Autodesk Inventor part; units mm, degrees
ref_plane "Work Plane1" through (47.9215, -19.8251, -5.5) normal (0, 0, 1) x (1, 0, 0)
ref_plane "Work Plane2" through (55.1914, -9.495, -5.5) normal (0, 0, 1) x (1, 0, 0)
ref_plane "YZ Plane" through (0, 0, 0) normal (1, 0, 0) x (0, 1, 0)
sketch "Sketch1" plane through (0, 0, 0) normal (0, 0, 1) x (1, 0, 0)
  circle A0 centre (66.3461, 11.6829) radius 1.35
  circle A1 centre (66.349, 28.6829) radius 1.35
  circle A2 centre (72.6461, 5.1829) radius 1.35
  circle A3 centre (72.649, 35.1829) radius 1.35
  line L0 (77.149, 32.3829) -> (77.149, 37.9829)
  line L1 (77.149, 7.9829) -> (77.149, 2.3829)
  line L2 (77.149, 32.3829) -> (69.149, 32.3829)
  line L3 (69.149, 32.3829) -> (69.149, 7.9829)
  line L4 (69.149, 7.9829) -> (77.149, 7.9829)
  circle A4 centre (16.149, 20.1829) radius 4.5
  line L5 (77.149, 37.9829) -> (52.149, 37.9829)
  arc A5 (14.1608, 31.0018) -> (14.1608, 9.3641) centre (16.149, 20.1829) ccw
  line L6 (52.149, 37.9829) -> (14.1608, 31.0018)
  line L7 (77.149, 2.3829) -> (52.149, 2.3829)
  line L8 (52.149, 2.3829) -> (14.1608, 9.3641)
  line L9 (63.549, 7.9829) -> (63.549, 32.3829)
  line L10 (63.549, 32.3829) -> (52.149, 32.3829)
  line L11 (52.149, 32.3829) -> (24.5301, 27.3073)
  line L12 (52.149, 7.9829) -> (63.549, 7.9829)
  line L13 (52.149, 7.9829) -> (24.5301, 13.0585)
  arc A6 (24.5301, 13.0585) -> (24.5301, 27.3073) centre (16.149, 20.1829) ccw
  point P0 (0, 0)
  dimension "d2" = 9
  dimension "d26" = 8
  dimension "d27" = 8
  dimension "d29" = 2.8
  dimension "d30" = 6.3
  dimension "d31" = 6.3
  dimension "d32" = 25
  dimension "d33" = 22
  dimension "d34" = 25
  dimension "d43" = 5.6
  dimension "d44" = 5.6
  dimension "d46" = 5.6
  dimension "d47" = 11.4
  dimension "d48" = 11.4
extrude "Extrusion1" add sketch "Sketch1" along normal blind 3
ref_plane "Work Plane1" through (47.9215, -19.8251, -5.5) normal (0, 0, 1) x (1, 0, 0)
sketch "Sketch5" plane through (0, 0, 0) normal (0, 0, -1) x (-1, 0, 0)
  line L0 (-52.149, 7.9829) -> (-63.549, 7.9829)
  line L1 (-63.549, 32.3829) -> (-52.149, 32.3829)
  circle A0 centre (-72.6461, 5.1829) radius 1.35
  circle A1 centre (-66.349, 28.6829) radius 1.35
  circle A2 centre (-66.3461, 11.6829) radius 1.35
  circle A3 centre (-72.649, 35.1829) radius 1.35
  line L2 (-77.149, 32.3829) -> (-77.149, 37.9829)
  line L3 (-77.149, 2.3829) -> (-77.149, 7.9829)
  line L4 (-77.149, 37.9829) -> (-52.149, 37.9829)
  line L5 (-77.149, 32.3829) -> (-69.149, 32.3829)
  line L6 (-69.149, 32.3829) -> (-69.149, 7.9829)
  line L7 (-69.149, 7.9829) -> (-77.149, 7.9829)
  line L8 (-77.149, 7.9829) -> (-77.149, 2.3829)
  line L9 (-77.149, 2.3829) -> (-52.149, 2.3829)
  line L10 (-52.149, 2.3829) -> (-52.149, 7.9829)
  line L11 (-63.549, 7.9829) -> (-63.549, 32.3829)
  line L12 (-52.149, 32.3829) -> (-52.149, 37.9829)
  line L13 (-63.549, 32.3829) -> (-52.149, 32.3829)
  line L14 (-52.149, 37.9829) -> (-77.149, 37.9829)
  line L15 (-77.149, 32.3829) -> (-77.149, 37.9829)
  circle A4 centre (-72.649, 35.1829) radius 1.35
  circle A5 centre (-66.349, 28.6829) radius 1.35
  circle A6 centre (-66.3461, 11.6829) radius 1.35
  circle A7 centre (-72.6461, 5.1829) radius 1.35
  point P0 (0, 0)
  dimension "d49" = 2.7
  dimension "d50" = 2.7
ref_plane "Work Plane2" through (55.1914, -9.495, -5.5) normal (0, 0, 1) x (1, 0, 0)
extrude "Extrusion5" add sketch "Sketch5" along normal up to surface (5.5 mm away)
sketch "Sketch6" plane through (52.149, 2.3829, 3) normal (0, -1, 0) x (1, 0, 0)
  line L0 (0, -3) -> (0, -8.5)
  line L1 (25, -8.5) -> (0, -8.5)
  line L2 (25, -8.5) -> (25, 0)
  line L3 (0, -3) -> (11.4, -8.5)
  line L4 (11.4, -8.5) -> (0, -8.5)
  line L5 (0, -8.5) -> (0, -3)
  line L6 (0, 0) -> (11.4, -5.5)
  line L7 (11.4, -8.5) -> (11.4, 0)
  line L8 (11.4, -5.5) -> (25, -5.5)
  line L9 (25, -8.5) -> (25, 0)
  line L10 (25, -5.5) -> (25, 0)
  line L11 (25, 0) -> (17, 0)
  line L12 (25, 0) -> (0, 0)
  point P0 (-52.149, -3)
extrude "Extrusion6" cut sketch "Sketch6" against normal through all contours L3 L1 L0 | L6 L12 L7 | L7 L12 L11 L2 L8
fillet "Fillet2" radius 3 4 edges at (63.549, 32.3829, -4) (24.5301, 27.3073, 1.5) (24.5301, 13.0585, 1.5) (63.549, 7.9829, -4)
sketch "Sketch7" plane through (0, 0, 3) normal (0, 0, 1) x (1, 0, 0)
  arc A0 (26.4411, 16.3006) -> (26.4411, 24.0653) centre (16.149, 20.1829) ccw
  circle A1 centre (16.149, 28.6829) radius 1
  point P0 (0, 0)
  dimension "d56" = 2
  dimension "d57" = 8.5
extrude "Extrusion7" cut sketch "Sketch7" against normal through all
pattern_circular "Circular Pattern1" count 8 over 360 about axis through (16.149, 20.1829, 0) along (0, 0, 1) of "Extrusion7"
properties part number "Arm" material "Aluminum-6061"
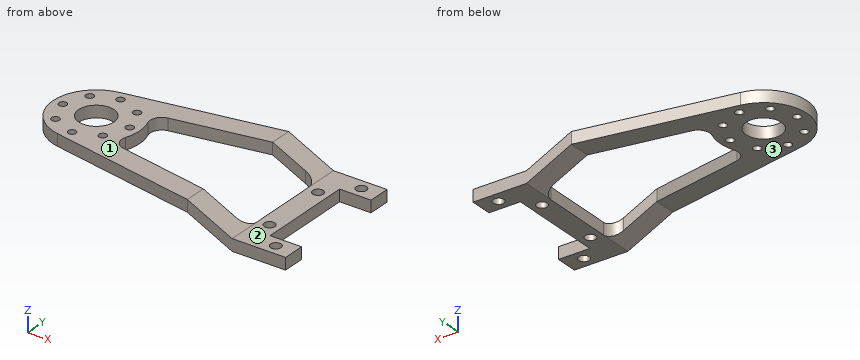
Check sheet for the modelled part. Datum: model origin and axes. Units: mm. Face numbers are marked on the shaded views. A direction names the side the tool comes from. Round coordinates to 2 decimals unless told otherwise and drop trailing zeros. Write each loop counter-clockwise with the first axis right and the second up, starting at its lowest first coordinate (ties: lowest second). Pieces come first, ordered by that corner, then holes. Notation, with made-up numbers: (82.5, 31.25) -> (102.5, 31.25) arc R14 ccw to (102.5, 36.25) -> close; hole circle Ø7 at (17.5, -26). An arc over 180 degrees is marked (long way). Put each result on its own line as item: value.
(1) Material ranges on line 1 (X direction, y = 20, z = 0.25); line 2 (Y direction, x = 49, z = 1.5); line 3 (X direction, y = 27, z = -4.75), recorded low to high.
Values found:
line 1: x = 5.15 to 6.67, 8.63 to 11.65, 20.65 to 23.67, 25.63 to 27.15
line 2: y = 2.96 to 8.56, 31.8 to 37.4
line 3: x = 63.55 to 69.15
(2) Sectioned sample at A-A (x = 43). Enter the section's corners in (y, z), plus the area to 3 significant figures.
Values found:
outline: (4.06, 0) -> (9.66, 0) -> (9.66, 3) -> (4.06, 3) -> close; (30.7, 0) -> (36.3, 0) -> (36.3, 3) -> (30.7, 3) -> close
area: 33.6 mm^2
(3) Go/stop test with flat-tipped pins: pin 1 Ø4 at (y, z) = (25, -1) entering from +X; pin 2 Ø3.5 at (x, y) = (72.65, 35.18) entering from +Z; pin 3 Ø12 at (x, y) = (45, 13) entering from -Z. Record where each tip stops, or that it passes through.
Values found:
pin 1: stops at x = 69.15
pin 2: stops at z = -2.5
pin 3: stops at z = 0
(4) Tool access check on the marked faces 1, 2 and 3. Record the directions out of +Z, -Z, +X, -X, +Y, -Y that give a thin tool (end or side, any length) a straight path to the whole face; none if there is none.
Values found:
face 1: +Z, +X, -X, +Y, -Y
face 2: +Z, +X, +Y, -Y
face 3: -Z, -X, +Y, -Y
